Could you check a few things on this drawing? It's one solid part, dimensions in mm from its lowest x, y, z. A direction names the side the tool comes from. Give positions to 0.01 mm unless a question says otherwise; leave off trailing zeros. Loops run counter-clockwise (first coordinate to the right, second up) from the corner with the lowest first, then second, coordinate; pieces in that order, holes last. Notation, with made-up numbers: (50.25, 59.25) - (83.25, 59.25) arc R20 ccw to (83.25, 93.25) - close; hole circle Ø2 at (-2.5, -13.75). An arc over 180 degrees is marked (long way). Answer as a JSON object with one key per item and string values.
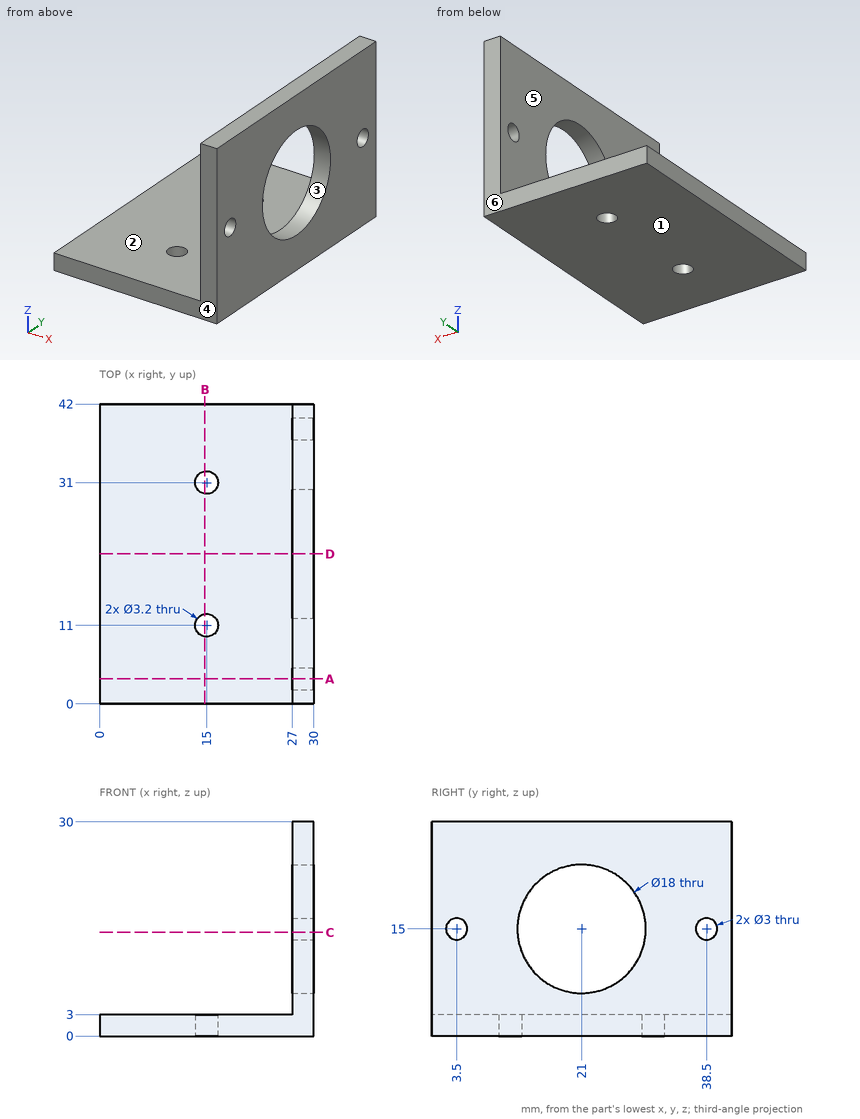
1) Imagine slicing it at A-A on y = 3.5. Write out the boundary of the cut face in (x, z), and give its area (3 significant figures).
Check sheet entries:
{"outline": "(0, 0) - (30, 0) - (30, 13.5) - (27, 13.5) - (27, 3) - (0, 3) - close; (27, 16.5) - (30, 16.5) - (30, 30) - (27, 30) - close", "area": "162 mm2"}
2) Imagine slicing it at D-D on y = 21. Write out the boundary of the cut face in (x, z).
Check sheet entries:
{"outline": "(0, 0) - (30, 0) - (30, 6) - (27, 6) - (27, 3) - (0, 3) - close; (27, 24) - (30, 24) - (30, 30) - (27, 30) - close"}
3) If we mould it in two halves opening along Y, with no side actions, what happens to the marked faces 3, 4, 5 and 6? For each: released by +Y, released by -Y, zero draft, split by the parting line, or undercut.
Check sheet entries:
{"face 3": "undercut", "face 4": "released by -Y", "face 5": "zero draft", "face 6": "released by +Y"}
4) I'm going to push flat-ended pins straight in: P1, Ø10, axis at x = 4.5, y = 23, coming from the -Z side; P2, Ø2, axis at x = 10, y = 9.5, coming from the +Z side; P3, Ø13.5, axis at y = 25, z = 20.5, coming from the -X side. Where does each tip first touch, or does it pass through?
Check sheet entries:
{"P1": "z = 0", "P2": "z = 3", "P3": "x = 27"}
5) I need wall thicknesses on L1, parallel to Y at x = 15, z = 1.4; L2, parallel to Z at x = 9, y = 22; L3, parallel to X at y = 40, z = 16.5. Which ranges of each line are inside material? Lowest first, please.
Check sheet entries:
{"L1": "0 to 9.4, 12.6 to 29.4, 32.6 to 42", "L2": "0 to 3", "L3": "27 to 30"}
6) Which directions (+Z, -Z, +X, -X, +Y, -Y) give clear straight access to the entire face, cutting with the end or side of a thin tool? Please do the marked faces 1 and 2.
Check sheet entries:
{"face 1": "-Z, +X, -X, +Y, -Y", "face 2": "+Z, -X, +Y, -Y"}
7) Imagine slicing it at C-C on z = 14.5. Write out the boundary of the cut face in (x, y), and give its area (3 significant figures).
Check sheet entries:
{"outline": "(27, 0) - (30, 0) - (30, 2.09) - (27, 2.09) - close; (27, 4.91) - (30, 4.91) - (30, 12.01) - (27, 12.01) - close; (27, 29.99) - (30, 29.99) - (30, 37.09) - (27, 37.09) - close; (27, 39.91) - (30, 39.91) - (30, 42) - (27, 42) - close", "area": "55.1 mm2"}
8) Imagine slicing it at B-B on x = 14.75. Write out the boundary of the cut face in (y, z), and give its area (3 significant figures).
Check sheet entries:
{"outline": "(0, 0) - (9.42, 0) - (9.42, 3) - (0, 3) - close; (12.58, 0) - (29.42, 0) - (29.42, 3) - (12.58, 3) - close; (32.58, 0) - (42, 0) - (42, 3) - (32.58, 3) - close", "area": "107 mm2"}
